Study the drawing (mm; zero at the part's minimum x, y, z) and answer. Coordinates: 2 decimals unless noted, no trailing zeros. Loops run counter-clockwise (first coordinate to the right, second up) from the corner with the lowest first, then second, coordinate; pieces in that order, holes last. Notation, with made-up numbers: (-26.75, -22) - (-12.75, -22) arc R34 ccw to (-12.75, 14) - close; hole circle Ø4 at (57.5, -13.5). An arc over 180 degrees is marked (long way). Write each question's results on one line, items separated by ' | '. Start each with the question number.
(1) Consider line 1 (Y direction, x = 50, z = 2.4); line 2 (Y direction, x = 47, z = 2.7); line 3 (Y direction, x = 31.5, z = 0.25). Determine where each line is inside the solid, lowest interval first. Write a range as from..to.
(2) Given pin 1 Ø1 at (x, z) = (65, 4) entering from -Y; pin 2 Ø2 at (x, z) = (78.5, 4) entering from +Y; pin 3 Ø2 at (x, z) = (55.5, 1.5) entering from +Y, each flat-ended and moving along its own axis, determine where each tip first touches the part or whether it passes through.
(3) Find section A-A on x = 50. Determine the outline of the cut face in (y, z).
(4) Find section B-B on y = 50. Determine the outline of the cut face in (x, z).
(5) Find section C-C on z = 3.6. Determine the outline of the cut face in (x, y).
(6) Find section D-D on y = 27.5. Determine the outline of the cut face in (x, z).
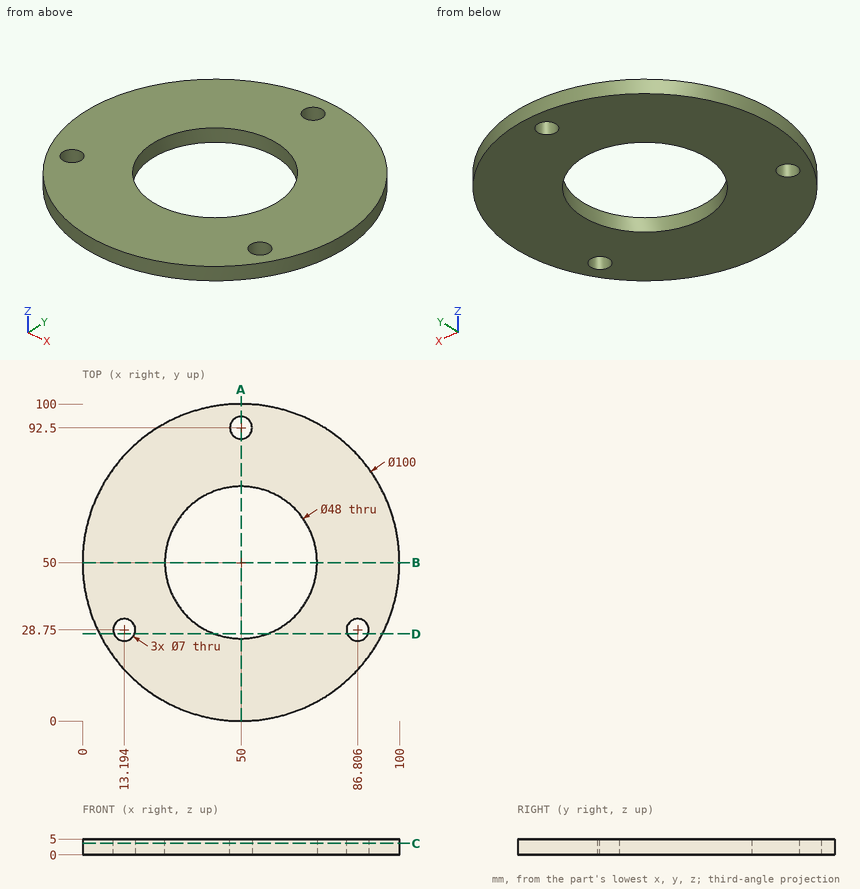
Values:
1) line 1: y = 0..26, 74..89, 96..100 | line 2: y = 0.09..26.19, 73.81..90.7, 94.3..99.91 | line 3: y = 3.55..34.71, 65.29..96.45
2) pin 1: stops at y = 2.15 | pin 2: stops at y = 91.76 | pin 3: stops at y = 99.8
3) outline: (0, 0) - (26, 0) - (26, 5) - (0, 5) - close; (74, 0) - (89, 0) - (89, 5) - (74, 5) - close; (96, 0) - (100, 0) - (100, 5) - (96, 5) - close
4) outline: (0, 0) - (26, 0) - (26, 5) - (0, 5) - close; (74, 0) - (100, 0) - (100, 5) - (74, 5) - close
5) outline: circle Ø100 at (50, 50); hole circle Ø7 at (13.19, 28.75); hole circle Ø48 at (50, 50); hole circle Ø7 at (50, 92.5); hole circle Ø7 at (86.81, 28.75)
6) outline: (5.35, 0) - (9.92, 0) - (9.92, 5) - (5.35, 5) - close; (16.46, 0) - (41.65, 0) - (41.65, 5) - (16.46, 5) - close; (58.35, 0) - (83.54, 0) - (83.54, 5) - (58.35, 5) - close; (90.08, 0) - (94.65, 0) - (94.65, 5) - (90.08, 5) - close
